```python
from build123d import *

# Parameters (mm, degrees)
RESSALTO_EXTRUS_O1_DEPTH = 10
ESBO_O3_R                = 2
CORTE_EXTRUS_O1_DEPTH    = 15
CHANFRO1_SIZE            = 1.6
FILETE1_R                = 0.5
FILETE2_R                = 0.94
RESSALTO_EXTRUS_O3_DEPTH = 10
CHANFRO5_SIZE            = 2
CHANFRO4_SIZE            = 1


with BuildPart() as part:
    # Esboço1 → Ressalto-extrusão1 (new body)
    with BuildSketch(Plane.XY):
        with BuildLine():
            Line((11, 14.25), (0.2, 14.25))
            Line((0.2, 14.25), (0.2, 11.25))
            Line((0.2, 11.25), (-5.8, 11.25))
            Line((-5.8, 11.25), (-5.8, -3.95))
            Line((-5.8, -3.95), (14.2, -3.95))
            Line((14.2, -3.95), (14.2, -8.95))
            Line((14.2, -8.95), (-10.8, -8.95))
            Line((-10.8, -8.95), (-10.8, 19.25))
            Line((-10.8, 19.25), (6, 19.25))
            Line((6, 19.25), (6, 16.25))
            Line((6, 16.25), (10.504380809, 16.25))
            ThreePointArc((10.504380809, 16.25), (10.676386068, 16.357306387), (10.826229508, 16.493861918))
            ThreePointArc((10.826229508, 16.493861918), (10.936214298, 16.519561844), (11, 16.426349589))
            Line((11, 16.426349589), (11, 16.25))
            Line((11, 16.25), (11, 14.25))
        make_face()
    extrude(amount=RESSALTO_EXTRUS_O1_DEPTH)

    # Esboço3 → Corte-extrusão1 (cut)
    with BuildSketch(Plane.XZ.offset(8.95)):
        with Locations(Location((6.2, 5, 0), (0, 0, 270))):
            Circle(ESBO_O3_R)
    extrude(amount=-CORTE_EXTRUS_O1_DEPTH, mode=Mode.SUBTRACT)

    # Chanfro1
    chanfro1_edges = [part.edges().sort_by_distance(p)[0] for p in [
        (6.2, -8.95, 7),
    ]]
    chamfer(chanfro1_edges, length=CHANFRO1_SIZE)

    # Filete1
    filete1_edges = [part.edges().sort_by_distance(p)[0] for p in [
        (6.2, -3.95, 7),
    ]]
    fillet(filete1_edges, radius=FILETE1_R)

    # Filete2
    filete2_edges = [part.edges().sort_by_distance(p)[0] for p in [
        (6, 16.25, 5),
    ]]
    fillet(filete2_edges, radius=FILETE2_R)

    # Esboço5 → Ressalto-extrusão3 (add)
    with BuildSketch(Plane.XY.offset(10)):
        Polygon((6, 19.25), (6, 21.25), (4, 21.25), (2, 19.25), align=None)
    extrude(amount=-RESSALTO_EXTRUS_O3_DEPTH)

    # Chanfro5
    chanfro5_edges = [part.edges().sort_by_distance(p)[0] for p in [
        (14.2, -8.95, 5),
        (-10.8, -8.95, 5),
        (-10.8, 19.25, 5),
    ]]
    chamfer(chanfro5_edges, length=CHANFRO5_SIZE)

    # Chanfro4
    chanfro4_edges = [part.edges().sort_by_distance(p)[0] for p in [
        (5.6, 14.25, 0),
        (0.2, 12.75, 0),
        (11, 14.25, 5),
        (0.2, 14.25, 5),
        (0.2, 12.75, 10),
        (-3.4, 19.25, 0),
        (-3.4, 19.25, 10),
        (3, 20.25, 10),
        (3, 20.25, 0),
        (14.2, -5.45, 0),
        (14.2, -5.45, 10),
        (1.7, -8.95, 0),
        (-10.8, 5.15, 0),
        (-9.8, 18.25, 0),
        (-9.8, -7.95, 0),
        (13.2, -7.95, 0),
        (1.7, -8.95, 10),
        (-10.8, 5.15, 10),
        (-9.8, 18.25, 10),
        (-9.8, -7.95, 10),
        (13.2, -7.95, 10),
        (5.6, 14.25, 10),
    ]]
    chamfer(chanfro4_edges, length=CHANFRO4_SIZE)


solid = part.part
```
Here's how the part is built. I have some questions about the finished solid (model axes, mm). A direction names the side the tool comes from. Give positions to 0.01 mm unless a question says otherwise; leave off trailing zeros. Loops run counter-clockwise (first coordinate to the right, second up) from the corner with the lowest first, then second, coordinate; pieces in that order, holes last. Notation, with made-up numbers: M 49,26.5 L 97,26.5 A19 cw 97,39.5 Z; hole C -23.75,8 d1. An arc over 180 degrees is marked long. Put each result on its own line as item: value. Start each with the question number.
(1) If we mould it in two halves opening along X, with no side actions, what happens to faces 1 (the flat face through (9, 16.25, 5)), 2 (the flat face through (3.59, 20.12, 9.51)), 3 (the flat face through (0.412, 14.066, 0.396))? For each: +X half, -X half, draft (parallel to the pull), parting line (faces both ways), or undercut.
(2) I want a section at A-A on x = -2.5. Please give me the cut outline in (y, z), then the cut area to 3 significant figures.
(3) I need wall thicknesses on line 1 along X through (y, z) = (-6.05, 5); line 2 along Y through (x, z) = (2, 7.25); line 3 along Y through (x, z) = (-4, 7.25). Which ranges of each line are inside material? Lowest first, please. Write a range as [from, to].
(4) I want a section at D-D on z = 9.5. Please give me the cut outline in (x, y), then the cut area to 3 significant figures.
(5) Will these pins go through, and if not, where does the flat tip stop? pin 1 Ø1 at (x, y) = (5.5, 14) entering from -Z; pin 2 Ø1.3 at (y, z) = (16, 3) entering from +X; pin 3 Ø1.8 at (x, z) = (9, 4) entering from +Y.
(6) For faces 4 (the flat face through (2, -3.95, 5)), 5 (the cylindrical face through (7.552, -5.92, 6.474)), 6 (the flat face through (0.384, 14.038, 9.604)), 7 (the flat face through (-9.47, 17.89, 0.51)), 8 (the flat face through (-0.3, 12.3, 0.5)), which set-ups out of +Z, -Z, +X, -X, +Y, -Y let a thin tool reach every point of the face, with its end or its side?
(7) I want a section at C-C on y = 4.5. Please give me the cut outline in (x, z), then the cut area to 3 significant figures.
Answer block:
1. face 1: undercut
1. face 2: -X half
1. face 3: +X half
2. outline: M -8.95,1 L -7.95,0 L -3.95,0 L -3.95,10 L -7.95,10 L -8.95,9 Z; M 11.25,0 L 18.25,0 L 19.25,1 L 19.25,9 L 18.25,10 L 11.25,10 Z
2. area: 128 mm^2
3. line 1: [-10.8, 4.2], [8.2, 14.2]
3. line 2: [-8.95, -3.95], [14.25, 19.25]
3. line 3: [-8.95, -3.95], [11.25, 19.25]
4. outline: M -10.3,-6.74 L -8.59,-8.45 L 11.99,-8.45 L 13.7,-6.74 L 13.7,-3.95 L -5.8,-3.95 L -5.8,11.25 L -0.3,11.25 L -0.3,13.25 L 1.2,14.75 L 10.5,14.75 L 11,15.25 L 11,16.43 A0.1 ccw 10.83,16.49 A1.12 cw 10.5,16.25 L 6.94,16.25 A0.94 cw 6,17.19 L 6,21.25 L 4.71,21.25 L 2.21,18.75 L -8.59,18.75 L -10.3,17.04 Z
4. area: 287 mm^2
5. pin 1: z = 0.75
5. pin 2: x = 11
5. pin 3: y = 16.25
6. face 4: +Z, -Z, +X
6. face 5: -Y
6. face 6: +Z, +X
6. face 7: -Z, -X, +Y
6. face 8: -Z, +X
7. outline: M -10.8,1 L -9.8,0 L -5.8,0 L -5.8,10 L -9.8,10 L -10.8,9 Z
7. area: 49.0 mm^2
